from build123d import *

# Parameters (mm, degrees)
SKETCH_R      = 12.25
SKETCH_R_2    = 2
SKETCH_R_3    = 4
PAD_DEPTH     = 12.5
SKETCH001_W   = 8
SKETCH001_H   = 40
PAD001_DEPTH  = 12.5
SKETCH002_W   = 8
SKETCH002_H   = 40
PAD002_DEPTH  = 12.5
SKETCH003_R   = 20.25
SKETCH003_R_2 = 12.25
SKETCH003_R_3 = 2
PAD003_DEPTH  = 12.5


with BuildPart() as part:
    # Sketch → Pad (new body, symmetric)
    with BuildSketch(Plane.YZ):
        Polygon((-49.7, 40), (49.7, 40), (49.7, 20), (66, 20), (66, -20), (49.7, -20), (49.7, -55.5), (-49.7, -55.5), (-49.7, -20), (-66, -20), (-66, 20), (-49.7, 20), align=None)
        Circle(SKETCH_R, mode=Mode.SUBTRACT)
        with Locations((-16.25, 0)):
            Circle(SKETCH_R_2, mode=Mode.SUBTRACT)
        with Locations((16.25, 0)):
            Circle(SKETCH_R_2, mode=Mode.SUBTRACT)
        with Locations((0, -38)):
            Circle(SKETCH_R_3, mode=Mode.SUBTRACT)
        with Locations((-30, -38)):
            Circle(SKETCH_R_3, mode=Mode.SUBTRACT)
        with Locations((30, -38)):
            Circle(SKETCH_R_3, mode=Mode.SUBTRACT)
    extrude(amount=PAD_DEPTH, both=True)

    # Sketch001 → Pad001 (join, symmetric)
    with BuildSketch(Plane.YZ):
        with Locations((-54, 0)):
            Rectangle(SKETCH001_W, SKETCH001_H)
    extrude(amount=PAD001_DEPTH, both=True)

    # Sketch002 → Pad002 (join, symmetric)
    with BuildSketch(Plane.YZ):
        with Locations((54, 0)):
            Rectangle(SKETCH002_W, SKETCH002_H)
    extrude(amount=PAD002_DEPTH, both=True)

    # Sketch003 → Pad003 (join, symmetric)
    with BuildSketch(Plane.YZ):
        Circle(SKETCH003_R)
        Circle(SKETCH003_R_2, mode=Mode.SUBTRACT)
        with Locations((-16.25, 0)):
            Circle(SKETCH003_R_3, mode=Mode.SUBTRACT)
        with Locations((16.25, 0)):
            Circle(SKETCH003_R_3, mode=Mode.SUBTRACT)
    extrude(amount=PAD003_DEPTH, both=True)


solid = part.part
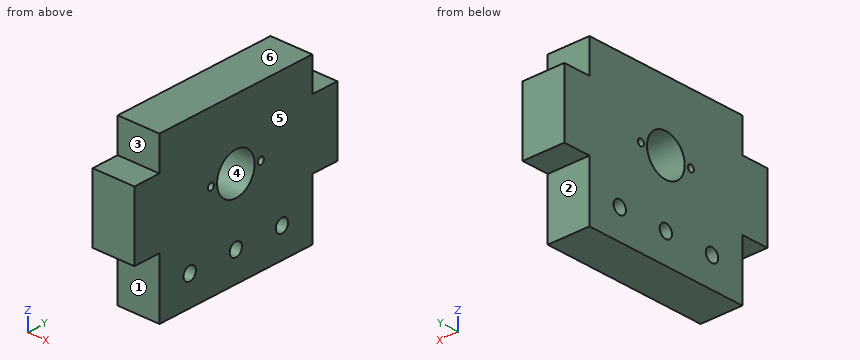
Can you work these out from the model? Positions are in its coordinate system, mm. Face numbers are marked on the shaded views. A direction names the side the tool comes from. Coordinates: 2 decimals unless noted, no trailing zeros. Loops run counter-clockwise (first coordinate to the right, second up) from the corner with the lowest first, then second, coordinate; pieces in that order, holes last. Notation, with made-up numbers: M 17.25,70.25 L 68.25,70.25 A10 cw 68.25,79.25 Z; hole C 24.25,47 d11. An arc over 180 degrees is marked long. Return JSON: item names as keys, results as strings. Group by question number.
Item 1: I'm going to push flat-ended pins straight in: pin 1 Ø5 at (x, y) = (5.5, 62) entering from +Z; pin 2 Ø13 at (x, y) = (4, 54.5) entering from -Z; pin 3 Ø6 at (x, z) = (-4, 33.5) entering from -Y; pin 4 Ø7.5 at (x, z) = (6, -41) entering from +Y. Where does each tip first touch, or does it pass through?
Item 2: Imagine slicing it at C-C (y = -30). Please give me the cut outline in (x, z).
Item 3: If I drill on L1, parallel to Z at x = -4.5, y = 0; L2, parallel to Z at x = 9.75, y = -60; L3, parallel to Y at x = 7.5, z = -42.5, over which ranges is the centre line in solid material (lowest first)? Write a range as from..to.
Item 4: Thinking about a two-plate mould opening in Z: for the marked faces 4, 5 and 6, which applies, released by +Z, released by -Z, zero draft, split by the parting line, or undercut?
Item 5: Imagine slicing it at D-D (x = 1.25). Please give me the cut outline in (y, z).
Item 6: Imagine slicing it at B-B (z = -38). Please give me the cut outline in (x, y), and give its area (4 significant figures).
Item 7: On a 3-axis mill with a long thin cutter (end or side, diameter ignored), from which of +Z, -Z, +X, -X, +Y, -Y can I reach the whole of each face in a straight line? I mean the marked faces 1, 2 and 3. Say none if no direction works.
Item 8: Imagine slicing it at A-A (y = 0). Please give me the cut outline in (x, z).
Verdict:
{
 "1": {"pin 1": "stops at z = 20", "pin 2": "stops at z = -55.5", "pin 3": "stops at y = -49.7", "pin 4": "stops at y = 49.7"},
 "2": {"outline": "M -12.5,-55.5 L 12.5,-55.5 L 12.5,-42 L -12.5,-42 Z; M -12.5,-34 L 12.5,-34 L 12.5,40 L -12.5,40 Z"},
 "3": {"L1": "z = -55.5..-42, -34..-12.25, 12.25..40", "L2": "z = -20..20", "L3": "y = -49.7..49.7"},
 "4": {"face 4": "undercut", "face 5": "zero draft", "face 6": "released by +Z"},
 "5": {"outline": "M -66,-20 L -49.7,-20 L -49.7,-55.5 L 49.7,-55.5 L 49.7,-20 L 66,-20 L 66,20 L 49.7,20 L 49.7,40 L -49.7,40 L -49.7,20 L -66,20 Z; hole C -30,-38 d8; hole C -16.25,0 d4; hole C 0,0 d24.5; hole C 0,-38 d8; hole C 16.25,0 d4; hole C 30,-38 d8"},
 "6": {"outline": "M -12.5,-49.7 L 12.5,-49.7 L 12.5,-34 L -12.5,-34 Z; M -12.5,-26 L 12.5,-26 L 12.5,-4 L -12.5,-4 Z; M -12.5,4 L 12.5,4 L 12.5,26 L -12.5,26 Z; M -12.5,34 L 12.5,34 L 12.5,49.7 L -12.5,49.7 Z", "area": "1,885 mm^2"},
 "7": {"face 1": "-Z, +X, -X, -Y", "face 2": "-Z, +X, -X, +Y", "face 3": "+Z, +X, -X, -Y"},
 "8": {"outline": "M -12.5,-55.5 L 12.5,-55.5 L 12.5,-42 L -12.5,-42 Z; M -12.5,-34 L 12.5,-34 L 12.5,-12.25 L -12.5,-12.25 Z; M -12.5,12.25 L 12.5,12.25 L 12.5,40 L -12.5,40 Z"}
}
